Geometry: final body of the model. Coordinates: model frame, mm. A direction names the side the tool comes from. Round coordinates to 2 decimals unless told otherwise and drop trailing zeros. Write each loop counter-clockwise with the first axis right and the second up, starting at its lowest first coordinate (ties: lowest second). Pieces come first, ordered by that corner, then holes. Notation, with made-up numbers: M 35.25,82.5 L 83.25,82.5 A24 ccw 83.25,97.5 Z; hole C -14,13 d7. An arc over 180 degrees is marked long. Use one line per item in the form item = value. Start each with the question number.
from build123d import *

# Parameters (mm, degrees)
SKETCH_1_W          = 80
SKETCH_1_H          = 100
EXTRUDE_1_DEPTH     = 5
SKETCH_3_W          = 5
SKETCH_3_H          = 100
EXTRUDE_2_DEPTH     = 100
SKETCH_4_R          = 2.25
SKETCH_4_R_2        = 17.5
CUT_EXTRUDE_1_DEPTH = 100
SKETCH_5_R          = 1.75
SKETCH_5_R_2        = 37.5
CUT_EXTRUDE_2_DEPTH = 22
FILLET_1_R          = 20


with BuildPart() as part:
    # 草图1 → 凸台-拉伸1 (new body)
    with BuildSketch(Plane(origin=(0, 0, 0), x_dir=(0, 0, -1), z_dir=(1, 0, 0))):
        Rectangle(SKETCH_1_W, SKETCH_1_H)
    extrude(amount=EXTRUDE_1_DEPTH)

    # 草图3 → 凸台-拉伸2 (add)
    with BuildSketch(Plane(origin=(5, 0, 0), x_dir=(0, 0, -1), z_dir=(1, 0, 0))):
        with Locations((37.5, 0)):
            Rectangle(SKETCH_3_W, SKETCH_3_H)
    extrude(amount=EXTRUDE_2_DEPTH)

    # 草图4 → 切除-拉伸1 (cut)
    with BuildSketch(Plane.ZY):
        with Locations((10, 21.75)):
            Circle(SKETCH_4_R)
        with Locations((26.661466638, 13.980630511)):
            Circle(SKETCH_4_R)
        with Locations(Location((-6.661466638, 13.980630511, 0), (0, 0, 180))):
            Circle(SKETCH_4_R)
        with Locations(Location((10, -21.75, 0), (0, 0, 180))):
            Circle(SKETCH_4_R)
        with Locations(Location((26.661466638, -13.980630511, 0), (0, 0, 180))):
            Circle(SKETCH_4_R)
        with Locations((-6.661466638, -13.980630511)):
            Circle(SKETCH_4_R)
        with Locations((10, 0)):
            Circle(SKETCH_4_R_2)
    extrude(amount=-CUT_EXTRUDE_1_DEPTH, mode=Mode.SUBTRACT)

    # 草图5 → 切除-拉伸2 (cut)
    with BuildSketch(Plane(origin=(0, 0, -40), x_dir=(-1, 0, 0), z_dir=(0, 0, -1))):
        with Locations(Location((-60, 42.5, 0), (0, 0, 90))):
            Circle(SKETCH_5_R)
        with Locations(Location((-29.9479618, 30.0520382, 0), (0, 0, 90))):
            Circle(SKETCH_5_R)
        with Locations(Location((-17.5, 0, 0), (0, 0, 90))):
            Circle(SKETCH_5_R)
        with Locations(Location((-29.9479618, -30.0520382, 0), (0, 0, 90))):
            Circle(SKETCH_5_R)
        with Locations(Location((-60, -42.5, 0), (0, 0, 90))):
            Circle(SKETCH_5_R)
        with Locations(Location((-90.0520382, -30.0520382, 0), (0, 0, 90))):
            Circle(SKETCH_5_R)
        with Locations(Location((-102.5, 0, 0), (0, 0, 90))):
            Circle(SKETCH_5_R)
        with Locations(Location((-90.0520382, 30.0520382, 0), (0, 0, 90))):
            Circle(SKETCH_5_R)
        with Locations(Location((-60, 0, 0), (0, 0, 90))):
            Circle(SKETCH_5_R_2)
    extrude(amount=-CUT_EXTRUDE_2_DEPTH, mode=Mode.SUBTRACT)

    # 圆角1
    fillet_1_edges = [part.edges().sort_by_distance(p)[0] for p in [
        (105, 50, -37.5),
        (105, -50, -37.5),
        (2.5, 50, 40),
        (2.5, -50, 40),
    ]]
    fillet(fillet_1_edges, radius=FILLET_1_R)


solid = part.part
1. Section query D-D (y = 21.75). Return loops of the section in (x, z), then the cut area to 3 significant figures.
2. Set-up query: faces 4 (the face through (21, -1, -35)), 5 (the face through (28.88, -31.44, -37.53)). Return all of +Z, -Z, +X, -X, +Y, -Y with unobstructed straight access to the full face (end or side cutting, diameter ignored); none if empty.
3. Contact query for flat-ended pins moving along their axis: pin 1 (5.5 mm diameter, centred on x = 29.95, y = 30.05, fed in from +Z); pin 2 (7 mm diameter, centred on y = 21.75, z = 10, fed in from +X); pin 3 (1 mm diameter, centred on y = -20, z = -15, fed in from -X). Output: stop coordinate, or through.
4. Ray query, probe 1 along Y at (x, z) = (3.7, 10); probe 2 along Z at (x, y) = (1.8, -21.75); probe 3 along Z at (x, y) = (10.5, 1). Return the intervals inside material, ascending.
5. Section query C-C (x = 17.5). Return loops of the section in (y, z).
6. Section query B-B (z = 10). Return loops of the section in (x, y).
7. Pull-direction query (X, two-part tool) for faces 1 (the face through (2.535, -44.297, 33.986)), 2 (the face through (59.33, -40.883, -37.535)), 3 (the face through (98.986, -44.297, -37.535)); classes: released by +X, released by -X, zero draft, split by the parting line, or undercut.
8. Section query A-A (x = 60). Return loops of the section in (y, z).
Checks:
q1.outline = M 0,-40 L 29.45,-40 L 29.45,-35 L 5,-35 L 5,7.75 L 0,7.75 Z; M 0,12.25 L 5,12.25 L 5,40 L 0,40 Z; M 90.55,-40 L 105,-40 L 105,-35 L 90.55,-35 Z
q1.area = 572 mm^2
q2.face_4 = +Z, +X, +Y, -Y
q2.face_5 = +Z, -Z
q3.pin_1 = -35
q3.pin_2 = 5
q3.pin_3 = 0
q4.probe_1 = -50 to -24, -19.5 to -17.5, 17.5 to 19.5, 24 to 50
q4.probe_2 = -40 to 7.75, 12.25 to 40
q4.probe_3 = -40 to -35
q5.outline = M -50,-40 L -1.75,-40 L -1.75,-35 L -50,-35 Z; M 1.75,-40 L 50,-40 L 50,-35 L 1.75,-35 Z
q6.outline = M 0,-50 L 5,-50 L 5,-24 L 0,-24 Z; M 0,-19.5 L 5,-19.5 L 5,-17.5 L 0,-17.5 Z; M 0,17.5 L 5,17.5 L 5,19.5 L 0,19.5 Z; M 0,24 L 5,24 L 5,50 L 0,50 Z
q7.face_1 = zero draft
q7.face_2 = undercut
q7.face_3 = released by +X
q8.outline = M -50,-40 L -44.25,-40 L -44.25,-35 L -50,-35 Z; M -40.75,-40 L -37.5,-40 L -37.5,-35 L -40.75,-35 Z; M 37.5,-40 L 40.75,-40 L 40.75,-35 L 37.5,-35 Z; M 44.25,-40 L 50,-40 L 50,-35 L 44.25,-35 Z
